Can you work these out from the model? Positions are in its coordinate system, mm. A direction names the side the tool comes from. Coordinates: 2 decimals unless noted, no trailing zeros. Write each loop counter-clockwise with the first axis right and the second up, starting at its lowest first coordinate (ties: lowest second). Pieces come first, ordered by that corner, then holes. Notation, with made-up numbers: (2, 54) - (34, 54) arc R22 ccw to (34, 85) - close; hole circle Ø4 at (47, 24.5). An arc over 180 degrees is marked (long way). Use one line per item in the form item = value. Start each with the question number.
(1) If we section it at B-B on z = 6: Please give me the cut outline in (x, y), then the cut area to 3 significant figures.
(2) For pin 1 Ø6 at (x, z) = (50.5, 6.5) entering from -Y; pin 2 Ø2.5 at (x, y) = (60, 20) entering from -Z; pin 3 Ø1.3 at (y, z) = (9.5, 12) entering from -X; pin 4 Ø1.2 at (y, z) = (20.5, 10) entering from -X, each with a flat end and sliding along its axis, tell me the tip position at first contact or that it passes through.
(3) On a 3-axis mill with a long thin cutter (end or side, diameter ignored), from which of +Z, -Z, +X, -X, +Y, -Y can I reach the whole of each face in a straight line? I mean faces 5 (the face through (42, 10, 9)), 6 (the face through (32.5, 20, 8)), 7 (the face through (38, 10, 9)). Say none if no direction works.
(4) If we section it at C-C on y = 12: Please give me the cut outline in (x, z), then the cut area to 3 significant figures.
(5) If we section it at A-A on y = 20: Please give me the cut outline in (x, z).
(6) Thinking about a two-plate mould opening in X: for faces 1 (the face through (18.89, 21.01, 1.48)), 2 (the face through (40, 30, 15)), 3 (the face through (48, 20, 14.5)), 4 (the face through (38, 30, 9)), which applies, pulls with the +X half, pulls with the -X half, needs draft (parallel to the pull), parting line crosses it, or undercut?
(7) If we section it at D-D on x = 46.5: Please give me the cut outline in (y, z).
(8) If I drill on probe 1 along X at (y, z) = (19.5, 10.75); probe 2 along Y at (x, z) = (20, 1.2); probe 3 along Z at (x, y) = (53, 23.5), over which ranges is the centre line in solid material (lowest first)? Write a range as from..to.
```python
from build123d import *

# Parameters (mm, degrees)
SKETCH_R      = 1.5
PAD_DEPTH     = 3
SKETCH001_W   = 4
SKETCH001_H   = 4.5
SKETCH001_W_2 = 4.5
SKETCH001_H_2 = 4
PAD001_DEPTH  = 12
CHAMFER_SIZE  = 1


with BuildPart() as part:
    # Sketch → Pad (new body)
    with BuildSketch(Plane.XY):
        with BuildLine():
            ThreePointArc((20, 26), (14, 20), (20, 14))
            Line((20, 14), (38, 8))
            Line((38, 8), (42, 8))
            Line((42, 8), (60, 14))
            ThreePointArc((60, 14), (66, 20), (60, 26))
            Line((42, 32), (60, 26))
            Line((38, 32), (42, 32))
            Line((20, 26), (38, 32))
        make_face()
        with Locations((20, 20)):
            Circle(SKETCH_R, mode=Mode.SUBTRACT)
        with Locations((60, 20)):
            Circle(SKETCH_R, mode=Mode.SUBTRACT)
    extrude(amount=PAD_DEPTH)

    # Sketch001 (on Face12 of Pad) → Pad001 (join)
    with BuildSketch(Plane.XY.offset(3)):
        with Locations((40, 29.75)):
            Rectangle(SKETCH001_W, SKETCH001_H)
        with Locations((40, 10.25)):
            Rectangle(SKETCH001_W, SKETCH001_H)
        with Locations((30.25, 20)):
            Rectangle(SKETCH001_W_2, SKETCH001_H_2)
        with Locations((49.75, 20)):
            Rectangle(SKETCH001_W_2, SKETCH001_H_2)
    extrude(amount=PAD001_DEPTH)

    # Chamfer
    chamfer_edges = [part.edges().sort_by_distance(p)[0] for p in [
        (32.5, 20, 15),
        (40, 12.5, 15),
        (40, 27.5, 15),
        (47.5, 20, 15),
    ]]
    chamfer(chamfer_edges, length=CHAMFER_SIZE)


solid = part.part
```
Reported:
q1.outline = (28, 18) - (32.5, 18) - (32.5, 22) - (28, 22) - close; (38, 8) - (42, 8) - (42, 12.5) - (38, 12.5) - close; (38, 27.5) - (42, 27.5) - (42, 32) - (38, 32) - close; (47.5, 18) - (52, 18) - (52, 22) - (47.5, 22) - close
q1.area = 72.0 mm2
q2.pin_1 = 18
q2.pin_2 = through
q2.pin_3 = 38
q2.pin_4 = 28
q3.face_5 = +Z, +X, +Y, -Y
q3.face_6 = +Z, +Y, -Y
q3.face_7 = +Z, -X, +Y, -Y
q4.outline = (26, 0) - (54, 0) - (54, 3) - (42, 3) - (42, 14.5) - (38, 14.5) - (38, 3) - (26, 3) - close
q4.area = 130 mm2
q5.outline = (14, 0) - (18.5, 0) - (18.5, 3) - (14, 3) - close; (21.5, 0) - (58.5, 0) - (58.5, 3) - (52, 3) - (52, 15) - (48.5, 15) - (47.5, 14) - (47.5, 3) - (32.5, 3) - (32.5, 14) - (31.5, 15) - (28, 15) - (28, 3) - (21.5, 3) - close; (61.5, 0) - (66, 0) - (66, 3) - (61.5, 3) - close
q6.face_1 = undercut
q6.face_2 = needs draft
q6.face_3 = undercut
q6.face_4 = pulls with the -X half
q7.outline = (9.5, 0) - (30.5, 0) - (30.5, 3) - (9.5, 3) - close
q8.probe_1 = 28..32.5, 47.5..52
q8.probe_2 = 14..18.5, 21.5..26
q8.probe_3 = 0..3
